For this review, take the finished solid that the model builds, in its own axes (mm). A direction names the side the tool comes from. Give positions to 0.01 mm unless a question says otherwise; leave off trailing zeros. Order: outer loops, then holes, each group sorted by start corner. A loop starts at its lowest first (then second) coordinate and runs counter-clockwise, first axis right, second up. Notation, with made-up numbers: (54, 33.5) - (85, 33.5) arc R8 ccw to (85, 39.5) - close; hole circle Ø1 at (62.25, 41). An arc over 180 degrees is marked (long way). Use a Markdown table: item, result. Add a question column.
1) Mouldability with a two-part tool opening along X and no side actions: class faces 1 (the face through (-3.616, 1.338, -0.084)), 2 (the face through (-20.14, 21.84, 3.63)), 3 (the face through (-10, 22, 0)) as released by +X, released by -X, zero draft, split by the parting line, or undercut.
2) We need section C-C on x = -13.5. Write out the cut boundary in (y, z), then the cut area to 3 significant figures.
3) Clearance check with flat-ended pins moving along their axes: P1, Ø2, axis at y = 12.5, z = -4.5, coming from the +X side; P2, Ø6, axis at y = 8.5, z = 0.5, coming from the -X side; P3, Ø6, axis at y = 13, z = -1.5, coming from the +X side. State where each tip first meets the part, or that it passes through.
4) Machinability: for faces 4 (the face through (-1.76, 0.27, 0.08)), 5 (the face through (-27, 15, 1)), which of the approach directions +Z, -Z, +X, -X, +Y, -Y give a long, thin tool a straight path to every point of the face, cutting with its end or side? Answer none if there is none.
5) Wall thickness on L1, parallel to Y at x = -5, z = -2.25; L2, parallel to Z at x = -8.5, y = 17.25; L3, parallel to X at y = 1.25, z = -4.25: over which ranges is each line inside the solid? List them lowest first.
6) We need section D-D on y = 1.5. Write out the cut boundary in (x, z), then the cut area to 3 significant figures.
7) We need section A-A on x = -5. Write out the cut boundary in (y, z), then the cut area to 3 significant figures.
8) We need section B-B on z = -0.75. Write out the cut boundary in (x, y), then the cut area to 3 significant figures.
```python
from build123d import *

# Parameters (mm, degrees)
SKETCH_1_R               = 3
EXTRUDE_1_DEPTH          = 6
CUT_EXTRUDE_1_DEPTH      = 39.88444419
CUT_EXTRUDE_3_DEPTH      = 20
CUT_EXTRUDE_4_DEPTH      = 3
CUT_EXTRUDE_5_DEPTH      = 39.884444283
CUT_EXTRUDE_5_DEPTH_BACK = 39.884444283


with BuildPart() as part:
    # Sketch 1 → Extrude 1 (new, symmetric)
    with BuildSketch(Plane.XY):
        with BuildLine():
            Line((-19.161323267, 0), (-3, 0))
            ThreePointArc((-3, 0), (-0.878679656, 0.878679656), (0, 3))
            Line((0, 3), (0, 24))
            Line((0, 24), (-30, 24))
            Line((-30, 24), (-30, 13.956143181))
            ThreePointArc((-30, 13.956143181), (-29.567922082, 12.405086708), (-28.396149212, 11.30081507))
            ThreePointArc((-28.396149212, 11.30081507), (-24.221365462, 7.661944199), (-22.125207826, 2.535900525))
            ThreePointArc((-22.125207826, 2.535900525), (-21.111669593, 0.720493647), (-19.161323267, 0))
        make_face()
        with Locations((-18, 4)):
            Circle(SKETCH_1_R, mode=Mode.SUBTRACT)
        with Locations((-5, 4)):
            Circle(SKETCH_1_R, mode=Mode.SUBTRACT)
    extrude(amount=EXTRUDE_1_DEPTH, both=True)

    # Sketch 2 → Cut-Extrude 1 (cut, through all)
    with BuildSketch(Plane.ZY.offset(30)):
        with BuildLine():
            ThreePointArc((0, 19.278746099), (-2, 17.278746099), (0, 15.278746099))
            Line((0, 15.278746099), (0, 19.278746099))
        make_face()
        with BuildLine():
            Line((0, 19.278746099), (0, 15.278746099))
            ThreePointArc((0, 15.278746099), (1.414213562, 15.864532537), (2, 17.278746099))
            ThreePointArc((2, 17.278746099), (1.414213562, 18.692959662), (0, 19.278746099))
        make_face()
    extrude(amount=-CUT_EXTRUDE_1_DEPTH, mode=Mode.SUBTRACT)

    # Sketch 2_4 → Cut-Extrude 3 (cut)
    with BuildSketch(Plane.ZY.offset(30)):
        Polygon((-3.25, 24), (-4, 19.746538635), (0, 19.746538635), (0, 24), align=None)
        Polygon((0, 19.746538635), (4, 19.746538635), (3.25, 24), (0, 24), align=None)
    extrude(amount=-CUT_EXTRUDE_3_DEPTH, mode=Mode.SUBTRACT)

    # Sketch 2_5 → Cut-Extrude 4 (cut)
    with BuildSketch(Plane.ZY.offset(30)):
        with BuildLine():
            Line((-3.324200633, 13.956143181), (0, 13.956143181))
            Line((0, 13.956143181), (0, 15.278746099))
            ThreePointArc((0, 15.278746099), (-2, 17.278746099), (0, 19.278746099))
            Line((0, 19.278746099), (0, 19.746538635))
            Line((0, 19.746538635), (-4, 19.746538635))
            ThreePointArc((-4, 19.746538635), (-4.668313251, 16.733905395), (-3.324200633, 13.956143181))
        make_face()
        with BuildLine():
            Line((0, 15.278746099), (0, 13.956143181))
            Line((0, 13.956143181), (3.324200633, 13.956143181))
            ThreePointArc((3.324200633, 13.956143181), (4.668313251, 16.733905395), (4, 19.746538635))
            Line((4, 19.746538635), (0, 19.746538635))
            Line((0, 19.746538635), (0, 19.278746099))
            ThreePointArc((0, 19.278746099), (1.414213562, 18.692959662), (2, 17.278746099))
            ThreePointArc((2, 17.278746099), (1.414213562, 15.864532537), (0, 15.278746099))
        make_face()
        with BuildLine():
            ThreePointArc((-3.324200633, 13.956143181), (-1.799133998, 12.936728497), (0, 12.578746099))
            Line((0, 12.578746099), (0, 13.956143181))
            Line((0, 13.956143181), (-3.324200633, 13.956143181))
        make_face()
        with BuildLine():
            Line((0, 13.956143181), (0, 12.578746099))
            ThreePointArc((0, 12.578746099), (1.799133998, 12.936728497), (3.324200633, 13.956143181))
            Line((3.324200633, 13.956143181), (0, 13.956143181))
        make_face()
    extrude(amount=-CUT_EXTRUDE_4_DEPTH, mode=Mode.SUBTRACT)

    # Sketch 3 → Cut-Extrude 5 (cut, two sides: drawn at the far end of the back side and taken through both)
    with BuildSketch(Plane(origin=(0, 24, 0), x_dir=(1, 0, 0), z_dir=(0, 1, 0)).offset(-CUT_EXTRUDE_5_DEPTH_BACK)):
        with BuildLine():
            Line((31.980847691, 73.421546804), (0, 6))
            ThreePointArc((0, 6), (-1.350889359, 0), (0, -6))
            Line((0, -6), (31.980847691, -73.421546804))
            Line((31.980847691, -73.421546804), (181.224803582, -73.421546804))
            Line((181.224803582, -73.421546804), (181.224803582, 73.421546804))
            Line((181.224803582, 73.421546804), (31.980847691, 73.421546804))
        make_face()
    extrude(amount=CUT_EXTRUDE_5_DEPTH + CUT_EXTRUDE_5_DEPTH_BACK, mode=Mode.SUBTRACT)


solid = part.part
```
Checked values:
| question | item | result |
|---|---|---|
| 1 | face 1 | undercut |
| 1 | face 2 | zero draft |
| 1 | face 3 | released by -X |
| 2 | outline | (0, -6) - (24, -6) - (24, -3.25) - (19.75, -4) - (19.75, 4) - (24, 3.25) - (24, 6) - (0, 6) - close; hole circle Ø4 at (17.28, 0) |
| 2 | area | 245 mm² |
| 3 | P1 | x = -0.23 |
| 3 | P2 | x = -28.72 |
| 3 | P3 | x = -0.61 |
| 4 | face 4 | +Z, -Z, +X, -Y |
| 4 | face 5 | -X |
| 5 | L1 | 0 to 1, 7 to 24 |
| 5 | L2 | -6 to -2, 2 to 6 |
| 5 | L3 | -21.6 to -19.2, -16.8 to -6.2, -3.8 to -0.69 |
| 6 | outline | (-21.76, -6) - (-19.66, -6) - (-19.66, 6) - (-21.76, 6) - close; (-16.34, -6) - (-6.66, -6) - (-6.66, 6) - (-16.34, 6) - close; (-3.34, -6) - (-0.4, -6) - (-0.4, -5.07) arc R14 cw to (-0.4, 5.07) - (-0.4, 6) - (-3.34, 6) - close |
| 6 | area | 170 mm² |
| 7 | outline | (0, -6) - (1, -6) - (1, 6) - (0, 6) - close; (7, -6) - (24, -6) - (24, 6) - (7, 6) - close; hole circle Ø4 at (17.28, 0) |
| 7 | area | 203 mm² |
| 8 | outline | (-29.7, 12.64) arc R3 ccw to (-28.4, 11.3) arc R12 cw to (-22.13, 2.54) arc R3 ccw to (-19.16, 0) - (-3, 0) arc R3 ccw to (-1.33, 0.51) - (-1.33, 15.42) - (-27, 15.42) - (-27, 12.64) - close; (-27, 19.13) - (-1.33, 19.13) - (-1.33, 24) - (-10, 24) - (-10, 19.75) - (-27, 19.75) - close; hole circle Ø6 at (-18, 4); hole circle Ø6 at (-5, 4) |
| 8 | area | 356 mm² |
